Here's how the part is built. I have some questions about the finished solid (model axes, mm). Face numbers are marked on the shaded views. A direction names the side the tool comes from. Give positions to 0.01 mm unless a question says otherwise; leave off trailing zeros. Write each loop counter-clockwise with the first axis right and the second up, starting at its lowest first coordinate (ties: lowest second). Pieces come first, ordered by that corner, then holes. Notation, with made-up numbers: M 13.5,27 L 70.5,27 A19 cw 70.5,39 Z; hole C 74,85.5 d1. An arc over 180 degrees is marked long. Use one line per item in the form item = value. Start each with the question number.
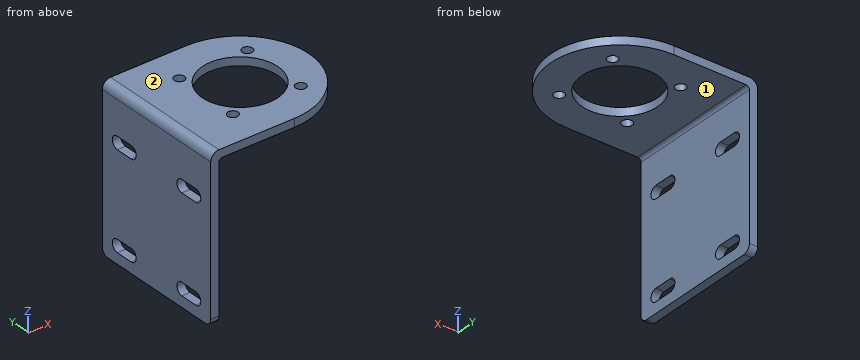
from build123d import *

# Parameters (mm, degrees)
SKETCH1_R           = 1.5
BOSS_EXTRUDE1_DEPTH = 2.4
SKETCH2_W           = 2.4
SKETCH2_H           = 40.1
BOSS_EXTRUDE2_DEPTH = 44.4
FILLET2_R           = 1
FILLET3_R           = 2.4
FILLET4_R           = 2
CUT_EXTRUDE1_DEPTH  = 45.4
SKETCH4_R           = 4
CUT_EXTRUDE2_DEPTH  = 2.4
SKETCH5_R           = 11
CUT_EXTRUDE3_DEPTH  = 2.4


with BuildPart() as part:
    # Sketch1 → Boss-Extrude1 (new body)
    with BuildSketch(Plane.XY):
        with BuildLine():
            Line((0, -20.05), (-24.35, -20.05))
            Line((-24.35, -20.05), (-24.35, 20.05))
            Line((-24.35, 20.05), (0, 20.05))
            ThreePointArc((0, 20.05), (20.05, 0), (0, -20.05))
        make_face()
        with Locations((-9.899494937, -9.899494937)):
            Circle(SKETCH1_R, mode=Mode.SUBTRACT)
        with Locations((-9.899494937, 9.899494937)):
            Circle(SKETCH1_R, mode=Mode.SUBTRACT)
        with Locations((9.899494937, 9.899494937)):
            Circle(SKETCH1_R, mode=Mode.SUBTRACT)
        with Locations((9.899494937, -9.899494937)):
            Circle(SKETCH1_R, mode=Mode.SUBTRACT)
    extrude(amount=BOSS_EXTRUDE1_DEPTH)

    # Sketch2 → Boss-Extrude2 (add)
    with BuildSketch(Plane(origin=(0, 0, 0), x_dir=(-1, 0, 0), z_dir=(0, 0, -1))):
        with Locations((23.15, 0)):
            Rectangle(SKETCH2_W, SKETCH2_H)
    extrude(amount=BOSS_EXTRUDE2_DEPTH)

    # Fillet2
    fillet2_edges = [part.edges().sort_by_distance(p)[0] for p in [
        (-21.95, 0, 0),
    ]]
    fillet(fillet2_edges, radius=FILLET2_R)

    # Fillet3
    fillet3_edges = [part.edges().sort_by_distance(p)[0] for p in [
        (-24.35, 0, 2.4),
    ]]
    fillet(fillet3_edges, radius=FILLET3_R)

    # Fillet4
    fillet4_edges = [part.edges().sort_by_distance(p)[0] for p in [
        (-23.15, 20.05, -44.4),
        (-23.15, -20.05, -44.4),
    ]]
    fillet(fillet4_edges, radius=FILLET4_R)

    # Sketch3 → Cut-Extrude1 (cut, through all)
    with BuildSketch(Plane.ZY.offset(24.35)):
        with BuildLine():
            Line((-41.27, 9.345), (-41.27, 14.545))
            ThreePointArc((-41.27, 14.545), (-39.445, 16.37), (-37.62, 14.545))
            Line((-37.62, 14.545), (-37.62, 9.345))
            ThreePointArc((-37.62, 9.345), (-39.445, 7.52), (-41.27, 9.345))
        make_face()
        with BuildLine():
            Line((-13.52, 9.345), (-13.52, 14.545))
            ThreePointArc((-13.52, 14.545), (-11.695, 16.37), (-9.87, 14.545))
            Line((-9.87, 14.545), (-9.87, 9.345))
            ThreePointArc((-9.87, 9.345), (-11.695, 7.52), (-13.52, 9.345))
        make_face()
        with BuildLine():
            Line((-41.27, -9.345), (-41.27, -14.545))
            ThreePointArc((-41.27, -14.545), (-39.445, -16.37), (-37.62, -14.545))
            Line((-37.62, -14.545), (-37.62, -9.345))
            ThreePointArc((-37.62, -9.345), (-39.445, -7.52), (-41.27, -9.345))
        make_face()
        with BuildLine():
            Line((-13.52, -9.345), (-13.52, -14.545))
            ThreePointArc((-13.52, -14.545), (-11.695, -16.37), (-9.87, -14.545))
            Line((-9.87, -14.545), (-9.87, -9.345))
            ThreePointArc((-9.87, -9.345), (-11.695, -7.52), (-13.52, -9.345))
        make_face()
    extrude(amount=-CUT_EXTRUDE1_DEPTH, mode=Mode.SUBTRACT)

    # Sketch4 → Cut-Extrude2 (cut)
    with BuildSketch(Plane.XY.offset(2.4)):
        Circle(SKETCH4_R)
    extrude(amount=-CUT_EXTRUDE2_DEPTH, mode=Mode.SUBTRACT)

    # Sketch5 → Cut-Extrude3 (cut)
    with BuildSketch(Plane.XY.offset(2.4)):
        Circle(SKETCH5_R)
    extrude(amount=-CUT_EXTRUDE3_DEPTH, mode=Mode.SUBTRACT)


solid = part.part
1) Suppose I cut it at A-A, the plane y = 0. List the corners of the cut face in (x, z) for me.
2) Suppose I cut it at D-D, the plane z = -21.5. List the corners of the cut face in (x, y) for me, and give its area (3 significant figures).
3) Please list where these lines run through material, in increasing order: line 1 (Y direction, x = 0, z = 0.75); line 2 (Z direction, x = -22, y = -8.5); line 3 (Z direction, x = 9.5, y = 12.5).
4) Suppose I cut it at C-C, the plane y = 13. List the corners of the cut face in (x, z) for me, and give its area (3 significant figures).
5) Will these pins go through, and if not, where does the flat tip stop? P1, Ø0.7, axis at x = -22.5, y = -11, coming from the +Z side; P2, Ø12, axis at y = 3, z = -32.5, coming from the +X side; P3, Ø2.5, axis at x = 9.9, y = 9.9, coming from the +Z side; P4, Ø12, axis at x = -9.5, y = 7.5, coming from the -Z side.
6) Suppose I cut it at B-B, the plane x = 2. List the corners of the cut face in (y, z) for me.
7) On a 3-axis mill with a long thin cutter (end or side, diameter ignored), from which of +Z, -Z, +X, -X, +Y, -Y can I reach the whole of each face in a straight line? I mean the marked faces 1 and 2. Say none if no direction works.
Checks:
q1.outline = M -24.35,-44.4 L -21.95,-44.4 L -21.95,-1 A1 cw -20.95,0 L -11,0 L -11,2.4 L -21.95,2.4 A2.4 ccw -24.35,0 Z; M 11,0 L 20.05,0 L 20.05,2.4 L 11,2.4 Z
q2.outline = M -24.35,-20.05 L -21.95,-20.05 L -21.95,20.05 L -24.35,20.05 Z
q2.area = 96.2 mm^2
q3.line_1 = -20.05 to -11, 11 to 20.05
q3.line_2 = -44.4 to -41.06, -37.83 to -13.31, -10.08 to 2.4
q3.line_3 = 0 to 2.4
q4.outline = M -24.35,-44.4 L -21.95,-44.4 L -21.95,-41.27 L -24.35,-41.27 Z; M -24.35,-37.62 L -21.95,-37.62 L -21.95,-13.52 L -24.35,-13.52 Z; M -24.35,-9.87 L -21.95,-9.87 L -21.95,-1 A1 cw -20.95,0 L 15.26,0 L 15.26,2.4 L -21.95,2.4 A2.4 ccw -24.35,0 Z
q4.area = 183 mm^2
q5.P1 = 2.39
q5.P2 = -21.95
q5.P3 = through
q5.P4 = 0
q6.outline = M -19.95,0 L -10.82,0 L -10.82,2.4 L -19.95,2.4 Z; M 10.82,0 L 19.95,0 L 19.95,2.4 L 10.82,2.4 Z
q7.face_1 = -Z, +X, +Y, -Y
q7.face_2 = +Z, +X, -X, +Y, -Y
